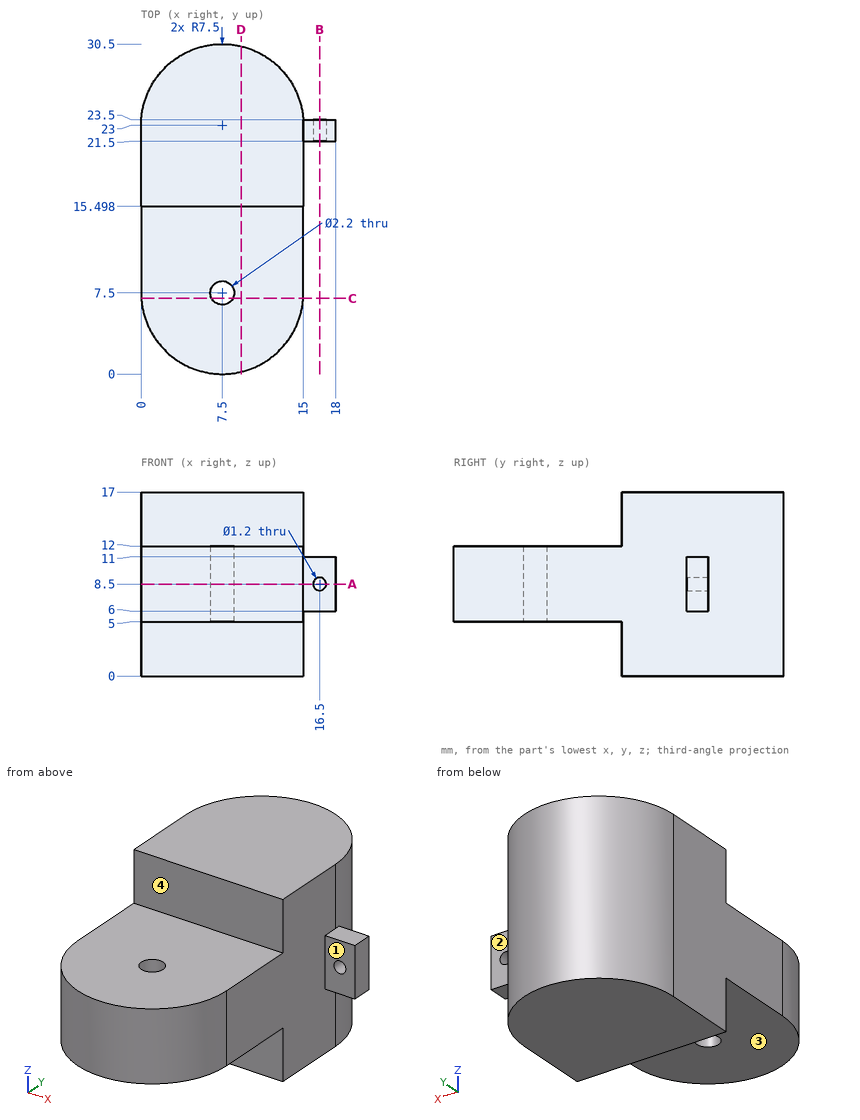
Could you check a few things on this drawing? It's one solid part, dimensions in mm from its lowest x, y, z. A direction names the side the tool comes from. Round coordinates to 2 decimals unless told otherwise and drop trailing zeros. Order: outer loops, then holes, each group sorted by start corner. A loop starts at its lowest first (then second) coordinate and runs counter-clockwise, first axis right, second up.
(1) Imagine slicing it at D-D (x = 9.25). Write out the boundary of the cut face in (y, z), plus the area to 3 significant figures.
Response values:
outline: (0.21, 5) - (15.5, 5) - (15.5, 0) - (30.29, 0) - (30.29, 17) - (15.5, 17) - (15.5, 12) - (0.21, 12) - close
area: 359 mm2
(2) Which directions (+Z, -Z, +X, -X, +Y, -Y) give clear straight access to the entire face, cutting with the end or side of a thin tool? Please do the marked faces 1, 2, 3 and 4.
Response values:
face 1: +Z, -Z, +X, -Y
face 2: +Z, -Z, +X, +Y
face 3: -Z, +X, -X, -Y
face 4: +Z, +X, -X, -Y
(3) Please list where these lines run through material, in increasing order: line 1 along X through (y, z) = (7.5, 9.5); line 2 along Y through (x, z) = (7.5, 8.5); line 3 along X through (y, z) = (22.35, 8.5).
Response values:
line 1: x = 0 to 6.4, 8.6 to 15
line 2: y = 0 to 6.4, 8.6 to 30.5
line 3: x = 0 to 15.9, 17.1 to 18
(4) Imagine slicing it at C-C (y = 7). Write out the boundary of the cut face in (x, z).
Response values:
outline: (0.02, 5) - (6.52, 5) - (6.52, 12) - (0.02, 12) - close; (8.48, 5) - (14.98, 5) - (14.98, 12) - (8.48, 12) - close
(5) Imagine slicing it at B-B (x = 16.5). Write out the boundary of the cut face in (y, z), plus the area to 3 significant figures.
Response values:
outline: (21.5, 6) - (23.5, 6) - (23.5, 7.9) - (21.5, 7.9) - close; (21.5, 9.1) - (23.5, 9.1) - (23.5, 11) - (21.5, 11) - close
area: 7.60 mm2
(6) Imagine slicing it at A-A (z = 8.5). Write out the boundary of the cut face in (x, y), plus the area to 3 significant figures.
Response values:
outline: (0, 7.5) arc R7.5 ccw to (15, 7.5) - (15, 21.5) - (15.9, 21.5) - (15.9, 23.5) - (14.98, 23.5) arc R7.5 ccw to (0, 23) - close; (17.1, 21.5) - (18, 21.5) - (18, 23.5) - (17.1, 23.5) - close; hole circle Ø2.2 at (7.5, 7.5)
area: 409 mm2
(7) I'm going to push flat-ended pins straight in: pin 1 (1.3 mm diameter, centred on x = 7.5, y = 7.5, fed in from -Z); pin 2 (5.5 mm diameter, centred on x = 5.5, z = 1.5, fed in from -Y); pin 3 (1.5 mm diameter, centred on x = 2, z = 5, fed in from -Y); pin 4 (10 mm diameter, centred on x = 4, z = 2.5, fed in from -Y). Where does each tip first touch, or does it pass through?
Response values:
pin 1: passes through
pin 2: stops at y = 15.5
pin 3: stops at y = 1.7
pin 4: stops at y = 0
